Build history of the part. All positions in model axes, mm. A direction names the side the tool comes from. Round coordinates to 2 decimals unless told otherwise and drop trailing zeros. Write each loop counter-clockwise with the first axis right and the second up, starting at its lowest first coordinate (ties: lowest second). Pieces come first, ordered by that corner, then holes. Notation, with made-up numbers: (59, 26) -> (101, 26) arc R24 cw to (101, 65) -> close; hole circle Ø1 at (43.5, -36.75). An arc over 180 degrees is marked (long way). Return JSON: item names as keys, results as strings.
from build123d import *

# Parameters (mm, degrees)
SKETCH1_R                    = 4.3688
BOSS_EXTRUDE1_DEPTH          = 3.175
EDGE_FLANGE1_STRIP_W         = 15.900000204
EDGE_FLANGE1_STRIP_H         = 3.175
EDGE_FLANGE1_STRIP_CUT_DEPTH = 21.59
EDGE_FLANGE1_DEPTH           = 21.59
EDGE_FLANGE1_FLAT_DEPTH      = 3.175


# Sheet-metal steps are written as plain solids
with BuildPart() as part:
    # Sketch1 → Boss-Extrude1 (new body)
    with BuildSketch(Plane.XY):
        Polygon((-10.795, 15.24), (10.795, 15.24), (10.795, -15.24), (-10.795, -15.24), (-10.795, -1.27), align=None)
        with Locations((0, 7.3025)):
            Circle(SKETCH1_R, mode=Mode.SUBTRACT)
    extrude(amount=BOSS_EXTRUDE1_DEPTH)

    # Edge-Flange1 strip (across the edge) → Edge-Flange1 strip cut (cut)
    with BuildSketch(Plane(origin=(10.795, -15.24, 0), x_dir=(0, 1, 0), z_dir=(-1, 0, 0))):
        with Locations((-3.175, -1.5875)):
            Rectangle(EDGE_FLANGE1_STRIP_W, EDGE_FLANGE1_STRIP_H)
    extrude(amount=EDGE_FLANGE1_STRIP_CUT_DEPTH, mode=Mode.SUBTRACT)

    # Edge-Flange1 bend section (across the edge) → Edge-Flange1 (add)
    with BuildSketch(Plane(origin=(10.795, -15.24, 0), x_dir=(0, 1, 0), z_dir=(-1, 0, 0))):
        with BuildLine():
            Line((0, 1.600000102), (3.175, 1.600000102))
            ThreePointArc((3.175, 1.600000102), (3.64362918, 0.46862918), (4.775000102, 0))
            Line((4.775000102, 0), (4.775000102, -3.175))
            ThreePointArc((4.775000102, -3.175), (1.39856515, -1.77643485), (0, 1.600000102))
        make_face()
    extrude(amount=EDGE_FLANGE1_DEPTH)

    # Edge-Flange1 profile (on flange) → Edge-Flange1 flat (add)
    with BuildSketch(Plane(origin=(0, -15.24, 0), x_dir=(1, 0, 0), z_dir=(0, 1, 0))):
        Polygon((-10.795, 1.600000102), (10.795, 1.600000102), (10.795, 13.335), (10.795, 34.925), (10.795, 43.815), (-10.795, 43.815), (-10.795, 34.925), (-10.795, 13.335), align=None)
    extrude(amount=EDGE_FLANGE1_FLAT_DEPTH)


solid = part.part
Q1. Saw through at C-C on x = 6.25. List the corners of the cut face in (y, z) (3 decimals), then the cut area to 3 significant figures.
Verdict:
{"outline": "(-15.24, -43.815) -> (-12.065, -43.815) -> (-12.065, -1.6) arc R1.6 cw to (-10.465, 0) -> (15.24, 0) -> (15.24, 3.175) -> (-10.465, 3.175) arc R4.775 ccw to (-15.24, -1.6) -> close", "area": "232 mm²"}
Q2. Saw through at A-A on x = 0. List the corners of the cut face in (y, z) (3 decimals).
Verdict:
{"outline": "(-15.24, -43.815) -> (-12.065, -43.815) -> (-12.065, -1.6) arc R1.6 cw to (-10.465, 0) -> (2.934, 0) -> (2.934, 3.175) -> (-10.465, 3.175) arc R4.775 ccw to (-15.24, -1.6) -> close; (11.671, 0) -> (15.24, 0) -> (15.24, 3.175) -> (11.671, 3.175) -> close"}
Q3. Saw through at B-B on y = 3.5. List the corners of the cut face in (x, z) (3 decimals), then the cut area to 3 significant figures.
Verdict:
{"outline": "(-10.795, 0) -> (-2.151, 0) -> (-2.151, 3.175) -> (-10.795, 3.175) -> close; (2.151, 0) -> (10.795, 0) -> (10.795, 3.175) -> (2.151, 3.175) -> close", "area": "54.9 mm²"}
Q4. 3-axis set-ups, long thin cutter, end or side, ignore diameter. For faces 1 (the flat face through (0, -14, -43.815)), 2 (the flat face through (0, -12.065, -23)): which of +Z, -Z, +X, -X, +Y, -Y reach the whole face in a straight line?
Verdict:
{"face 1": "-Z, +X, -X, +Y, -Y", "face 2": "-Z, +X, -X, +Y"}
Q5. Pin check, flat tips, straight feed: pin 1 Ø1.5 at (x, y) = (-3.5, -6.5) entering from -Z; pin 2 Ø8 at (x, z) = (6, -5.5) entering from +Y. Stop position of each tip, or through.
Verdict:
{"pin 1": "stops at z = 0", "pin 2": "stops at y = -12.06"}
Q6. Wall check: L1, parallel to Y at x = 6.5, z = -6 (3 decimals); L2, parallel to Z at x = 8.25, y = -1 (3 decimals); L3, parallel to Y at x = 0, z = 1.05. Give the ranges that are in metal, low to high.
Verdict:
{"L1": "y = -15.24 to -12.065", "L2": "z = 0 to 3.175", "L3": "y = -14.44 to 2.93, 11.67 to 15.24"}
Q7. Saw through at D-D on x = -3.25. List the corners of the cut face in (y, z) (3 decimals).
Verdict:
{"outline": "(-15.24, -43.815) -> (-12.065, -43.815) -> (-12.065, -1.6) arc R1.6 cw to (-10.465, 0) -> (4.383, 0) -> (4.383, 3.175) -> (-10.465, 3.175) arc R4.775 ccw to (-15.24, -1.6) -> close; (10.222, 0) -> (15.24, 0) -> (15.24, 3.175) -> (10.222, 3.175) -> close"}
